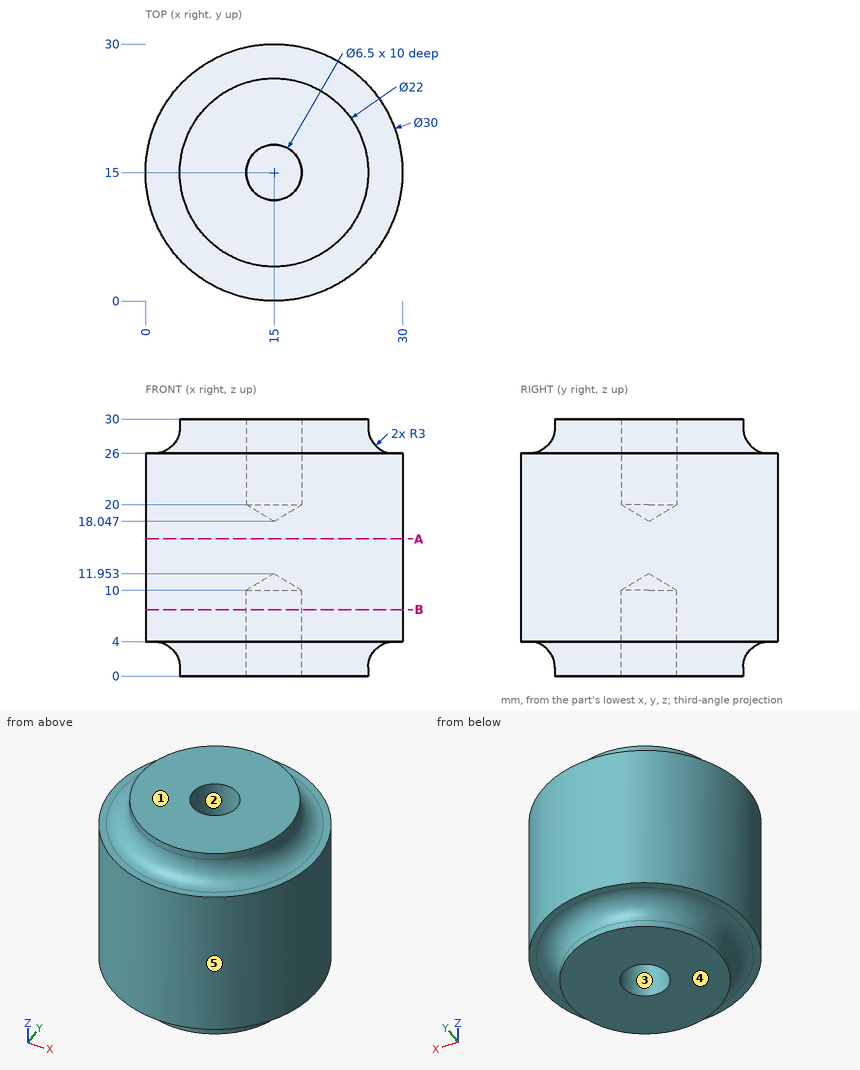
Source: three-view drawing plus pictorial views. Frame: mm from the lowest corner of the part. A direction names the side the tool comes from. Round coordinates to 2 decimals unless told otherwise and drop trailing zeros. Order: outer loops, then holes, each group sorted by start corner. A loop starts at its lowest first (then second) coordinate and runs counter-clockwise, first axis right, second up. Notation, with made-up numbers: (55.25, -7) - (76.25, -7) arc R13 ccw to (76.25, 14) - close; hole circle Ø5 at (-0.5, 60). An arc over 180 degrees is marked (long way). Write each question's results on one line, items separated by ' | '.
Item 1: Section B-B, the plane z = 7.75. Return the cut outline in (x, y), and give its area (3 significant figures).
Completed:
outline: circle Ø30 at (15, 15); hole circle Ø6.5 at (15, 15) | area: 674 mm^2
Item 2: First-contact query: pin 1 Ø4 at (x, y) = (15, 15) entering from +Z; pin 2 Ø4 at (y, z) = (22, 16) entering from -X; pin 3 Ø4 at (x, z) = (23, 18.5) entering from -Y. Flat tips, straight axial feed; report the tip coordinate or a pass-through.
Completed:
pin 1: z = 19.25 | pin 2: x = 0.86 | pin 3: y = 1.25
Item 3: Material intervals for line 1 along Y through (x, z) = (15, 7.5); line 2 along Z through (x, y) = (6, 4.5) (1 decimal); line 3 along Y through (x, z) = (13.5, 21.5) (1 decimal), sorted ascending. Write a range as [from, to].
Completed:
line 1: [0, 11.75], [18.25, 30] | line 2: [4, 26] | line 3: [0.1, 12.1], [17.9, 29.9]
Item 4: Section A-A, the plane z = 16. Return the cut outline in (x, y), and give its area (3 significant figures).
Completed:
outline: circle Ø30 at (15, 15) | area: 707 mm^2
Item 5: Mould query, pull axis Y, two halves, no side actions, for the marked faces 3, 4 and 5. Classes: pulls with the +Y half, pulls with the -Y half, needs draft (parallel to the pull), parting line crosses it, or undercut.
Completed:
face 3: undercut | face 4: needs draft | face 5: parting line crosses it
Item 6: Reachability of the marked faces 1 and 2 from +Z, -Z, +X, -X, +Y, -Y: full face, straight path, thin tool, end or side. Return the list, or none.
Completed:
face 1: +Z, +X, -X, +Y, -Y | face 2: +Z
